Work out the finished part from the listing and answer in its coordinate system (mm). Round coordinates to 2 decimals unless told otherwise and drop trailing zeros. Write each loop counter-clockwise with the first axis right and the second up, starting at its lowest first coordinate (ties: lowest second). Pieces come first, ordered by that corner, then holes. Notation, with made-up numbers: (64.25, 15.5) - (77.25, 15.5) arc R10 cw to (77.25, 25.5) - close; hole circle Ø5 at (3, 0). An arc over 180 degrees is marked (long way). Answer as a JSON object with one key per item and string values.
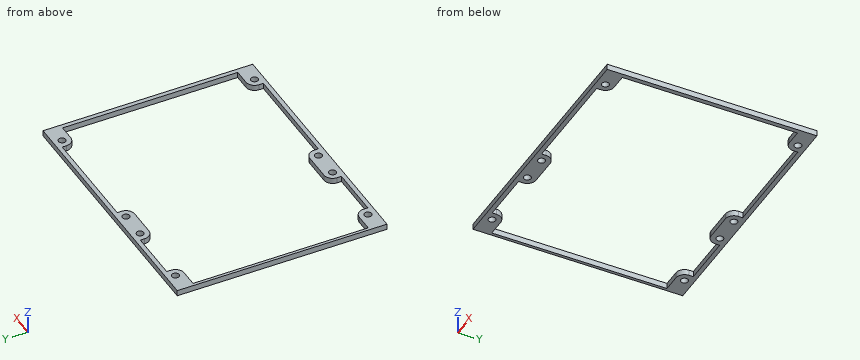
```python
from build123d import *

# Parameters (mm, degrees)
SKETCH2_W           = 180.5
SKETCH2_H           = 145.5
BOSS_EXTRUDE1_DEPTH = 4
CUT_EXTRUDE2_REACH  = 6
SKETCH5_R           = 2.5


with BuildPart() as part:
    # Sketch2 → Boss-Extrude1 (new body)
    with BuildSketch(Plane.XY):
        Rectangle(SKETCH2_W, SKETCH2_H)
    extrude(amount=BOSS_EXTRUDE1_DEPTH)

    # Sketch5 → Cut-Extrude2 (cut, up to next)
    with BuildSketch(Plane.XY.offset(4), mode=Mode.PRIVATE) as cut_extrude2_sk1:
        with Locations((-76.25, 66.75)):
            Circle(SKETCH5_R)
    cut_extrude2_tool1 = extrude(cut_extrude2_sk1.sketch, amount=-CUT_EXTRUDE2_REACH, mode=Mode.PRIVATE) & part.part
    add(cut_extrude2_tool1.solids().sort_by_distance((-76.25, 66.75, 4))[0], mode=Mode.SUBTRACT)
    # Sketch5 → Cut-Extrude2 (cut, up to next)
    with BuildSketch(Plane.XY.offset(4), mode=Mode.PRIVATE) as cut_extrude2_sk2:
        with Locations((-28.75, 66.75)):
            Circle(SKETCH5_R)
    cut_extrude2_tool2 = extrude(cut_extrude2_sk2.sketch, amount=-CUT_EXTRUDE2_REACH, mode=Mode.PRIVATE) & part.part
    add(cut_extrude2_tool2.solids().sort_by_distance((-28.75, 66.75, 4))[0], mode=Mode.SUBTRACT)
    # Sketch5 → Cut-Extrude2 (cut, up to next)
    with BuildSketch(Plane.XY.offset(4), mode=Mode.PRIVATE) as cut_extrude2_sk3:
        with Locations((-9.75, 66.75)):
            Circle(SKETCH5_R)
    cut_extrude2_tool3 = extrude(cut_extrude2_sk3.sketch, amount=-CUT_EXTRUDE2_REACH, mode=Mode.PRIVATE) & part.part
    add(cut_extrude2_tool3.solids().sort_by_distance((-9.75, 66.75, 4))[0], mode=Mode.SUBTRACT)
    # Sketch5 → Cut-Extrude2 (cut, up to next)
    with BuildSketch(Plane.XY.offset(4), mode=Mode.PRIVATE) as cut_extrude2_sk4:
        with Locations((76.25, 66.75)):
            Circle(SKETCH5_R)
    cut_extrude2_tool4 = extrude(cut_extrude2_sk4.sketch, amount=-CUT_EXTRUDE2_REACH, mode=Mode.PRIVATE) & part.part
    add(cut_extrude2_tool4.solids().sort_by_distance((76.25, 66.75, 4))[0], mode=Mode.SUBTRACT)
    # Sketch5 → Cut-Extrude2 (cut, up to next)
    with BuildSketch(Plane.XY.offset(4), mode=Mode.PRIVATE) as cut_extrude2_sk5:
        with Locations((76.25, -66.75)):
            Circle(SKETCH5_R)
    cut_extrude2_tool5 = extrude(cut_extrude2_sk5.sketch, amount=-CUT_EXTRUDE2_REACH, mode=Mode.PRIVATE) & part.part
    add(cut_extrude2_tool5.solids().sort_by_distance((76.25, -66.75, 4))[0], mode=Mode.SUBTRACT)
    # Sketch5 → Cut-Extrude2 (cut, up to next)
    with BuildSketch(Plane.XY.offset(4), mode=Mode.PRIVATE) as cut_extrude2_sk6:
        with Locations((-9.75, -66.75)):
            Circle(SKETCH5_R)
    cut_extrude2_tool6 = extrude(cut_extrude2_sk6.sketch, amount=-CUT_EXTRUDE2_REACH, mode=Mode.PRIVATE) & part.part
    add(cut_extrude2_tool6.solids().sort_by_distance((-9.75, -66.75, 4))[0], mode=Mode.SUBTRACT)
    # Sketch5 → Cut-Extrude2 (cut, up to next)
    with BuildSketch(Plane.XY.offset(4), mode=Mode.PRIVATE) as cut_extrude2_sk7:
        with Locations((-28.75, -66.75)):
            Circle(SKETCH5_R)
    cut_extrude2_tool7 = extrude(cut_extrude2_sk7.sketch, amount=-CUT_EXTRUDE2_REACH, mode=Mode.PRIVATE) & part.part
    add(cut_extrude2_tool7.solids().sort_by_distance((-28.75, -66.75, 4))[0], mode=Mode.SUBTRACT)
    # Sketch5 → Cut-Extrude2 (cut, up to next)
    with BuildSketch(Plane.XY.offset(4), mode=Mode.PRIVATE) as cut_extrude2_sk8:
        with Locations((-76.25, -66.75)):
            Circle(SKETCH5_R)
    cut_extrude2_tool8 = extrude(cut_extrude2_sk8.sketch, amount=-CUT_EXTRUDE2_REACH, mode=Mode.PRIVATE) & part.part
    add(cut_extrude2_tool8.solids().sort_by_distance((-76.25, -66.75, 4))[0], mode=Mode.SUBTRACT)
    # Sketch5 → Cut-Extrude2 (cut, up to next)
    with BuildSketch(Plane.XY.offset(4), mode=Mode.PRIVATE) as cut_extrude2_sk9:
        with BuildLine():
            Line((-70.25, 69.75), (-34.75, 69.75))
            Line((-34.75, 69.75), (-34.75, 66.75))
            ThreePointArc((-34.75, 66.75), (-32.992640687, 62.507359313), (-28.75, 60.75))
            Line((-28.75, 60.75), (-9.75, 60.75))
            ThreePointArc((-9.75, 60.75), (-5.507359313, 62.507359313), (-3.75, 66.75))
            Line((-3.75, 66.75), (-3.75, 69.75))
            Line((-3.75, 69.75), (70.25, 69.75))
            Line((70.25, 69.75), (70.25, 66.75))
            ThreePointArc((70.25, 66.75), (72.007359313, 62.507359313), (76.25, 60.75))
            Line((76.25, 60.75), (87.25, 60.75))
            Line((87.25, 60.75), (87.25, -60.75))
            Line((87.25, -60.75), (76.25, -60.75))
            ThreePointArc((76.25, -60.75), (72.007359313, -62.507359313), (70.25, -66.75))
            Line((70.25, -66.75), (70.25, -69.75))
            Line((70.25, -69.75), (-3.75, -69.75))
            Line((-3.75, -69.75), (-3.75, -66.75))
            ThreePointArc((-3.75, -66.75), (-5.507359313, -62.507359313), (-9.75, -60.75))
            Line((-9.75, -60.75), (-28.75, -60.75))
            ThreePointArc((-28.75, -60.75), (-32.992640687, -62.507359313), (-34.75, -66.75))
            Line((-34.75, -66.75), (-34.75, -69.75))
            Line((-34.75, -69.75), (-70.25, -69.75))
            Line((-70.25, -69.75), (-70.25, -66.75))
            ThreePointArc((-70.25, -66.75), (-72.007359313, -62.507359313), (-76.25, -60.75))
            Line((-76.25, -60.75), (-88.25, -60.75))
            Line((-88.25, -60.75), (-88.25, 60.75))
            Line((-88.25, 60.75), (-76.25, 60.75))
            ThreePointArc((-76.25, 60.75), (-72.007359313, 62.507359313), (-70.25, 66.75))
            Line((-70.25, 66.75), (-70.25, 69.75))
        make_face()
    cut_extrude2_tool9 = extrude(cut_extrude2_sk9.sketch, amount=-CUT_EXTRUDE2_REACH, mode=Mode.PRIVATE) & part.part
    add(cut_extrude2_tool9.solids().sort_by_distance((-0.02205, 0, 4))[0], mode=Mode.SUBTRACT)


solid = part.part
```
Item 1: A cutting plane is placed at B-B (x = -16.5). Write down the section's boundary in (y, z).
Results found:
{"outline": "(-72.75, 0) - (-60.75, 0) - (-60.75, 4) - (-72.75, 4) - close; (60.75, 0) - (72.75, 0) - (72.75, 4) - (60.75, 4) - close"}
Item 2: This flat-tipped pin is pushed along its axis until it touches: P1, Ø4.5, axis at x = -28.75, y = 66.75, coming from the +Z side. Where does it stop, or does it pass through?
Results found:
{"P1": "through"}
Item 3: A cutting plane is placed at C-C (z = 2.9). Give the number of separate pieces and of enclosed holes in the cut face, and give its area (3 significant figures).
Results found:
{"separate pieces": "1", "enclosed holes": "9", "area": "2,750 mm²"}
Item 4: Consider line 1 along Y through (x, z) = (-76.25, 1.5); line 2 along Y through (x, z) = (52.5, 0.8); line 3 along X through (y, z) = (0, 2.3). Determine where each line is inside the solid, lowest interval first.
Results found:
{"line 1": "-72.75 to -69.25, -64.25 to -60.75, 60.75 to 64.25, 69.25 to 72.75", "line 2": "-72.75 to -69.75, 69.75 to 72.75", "line 3": "-90.25 to -88.25, 87.25 to 90.25"}
Item 5: A cutting plane is placed at A-A (y = 22.5). Write down the section's boundary in (x, z), and give its area (3 significant figures).
Results found:
{"outline": "(-90.25, 0) - (-88.25, 0) - (-88.25, 4) - (-90.25, 4) - close; (87.25, 0) - (90.25, 0) - (90.25, 4) - (87.25, 4) - close", "area": "20.0 mm²"}
